Could you check a few things on this model? Use its own coordinates, in mm. Coordinates: 2 decimals unless noted, no trailing zeros. Loops run counter-clockwise (first coordinate to the right, second up) from the corner with the lowest first, then second, coordinate; pieces in that order, holes last.
from build123d import *

# Parameters (mm, degrees)
CYLINDER001_R     = 0.325
CYLINDER001_DEPTH = 10
CYLINDER002_R     = 0.325
CYLINDER002_DEPTH = 10
CYLINDER_R        = 3.75
CYLINDER_DEPTH    = 9.5


with BuildPart() as obj1:
    # Cylinder001 → Cylinder001 (new body)
    with BuildSketch(Plane(origin=(-9, 0, -10), x_dir=(1, 0, 0), z_dir=(0, 0, 1))):
        Circle(CYLINDER001_R)
    extrude(amount=CYLINDER001_DEPTH)


with BuildPart() as fusion:
    # Cone → Cone (revolve)
    with BuildSketch(Plane(origin=(-9, 0, 0), x_dir=(1, 0, 0), z_dir=(0, -1, 0))):
        Polygon((0, 0), (0.325, 0), (1.25, 3), (0, 3), align=None)
    revolve(axis=Axis((-9, 0, 0), (0, 0, 1)))

    # Fusion: union obj1
    add(obj1.part)


with BuildPart() as fusion_1:
    # Fusion placement: moved
    add(fusion.part.moved(Location((10.5, 0, -3))))


with BuildPart() as obj2:
    # Cylinder002 → Cylinder002 (new body)
    with BuildSketch(Plane(origin=(-9, 0, -10), x_dir=(1, 0, 0), z_dir=(0, 0, 1))):
        Circle(CYLINDER002_R)
    extrude(amount=CYLINDER002_DEPTH)


with BuildPart() as fusion001:
    # Cone001 → Cone001 (revolve)
    with BuildSketch(Plane(origin=(-9, 0, 0), x_dir=(1, 0, 0), z_dir=(0, -1, 0))):
        Polygon((0, 0), (0.325, 0), (1.25, 3), (0, 3), align=None)
    revolve(axis=Axis((-9, 0, 0), (0, 0, 1)))

    # Fusion001: union obj2
    add(obj2.part)


with BuildPart() as fusion001_1:
    # Fusion001 placement: moved
    add(fusion001.part.moved(Location((7.5, 0, -3))))


with BuildPart() as fusion002:
    # Cylinder → Cylinder (new body)
    with BuildSketch(Plane.XY):
        Circle(CYLINDER_R)
    extrude(amount=CYLINDER_DEPTH)

    # Fusion002: union Fusion, Fusion001
    add(fusion_1.part)
    add(fusion001_1.part)


solid = fusion002.part
(1) Imagine slicing it at C-C, the plane x = -1.5. Write out the boundary of the cut face in (y, z) (3 decimals).
Answers:
outline: (-3.437, 0) - (-1.25, 0) - (-0.325, -3) - (-0.325, -13) - (0.325, -13) - (0.325, -3) - (1.25, 0) - (3.437, 0) - (3.437, 9.5) - (-3.437, 9.5) - close
(2) For pin 1 (3 mm diameter, centred on x = -2.5, z = 0.5, fed in from +Y); pin 2 (1 mm diameter, centred on x = -1.5, z = 0.5, fed in from -Y), each with a flat end and sliding along its axis, tell me the tip position at first contact or that it passes through.
Answers:
pin 1: stops at y = 3.61
pin 2: stops at y = -3.61
(3) Imagine slicing it at A-A, the plane y = 0. Write out the boundary of the cut face in (x, z) (3 decimals), and give its area (3 significant figures).
Answers:
outline: (-3.75, 0) - (-2.75, 0) - (-1.825, -3) - (-1.825, -13) - (-1.175, -13) - (-1.175, -3) - (-0.25, 0) - (0.25, 0) - (1.175, -3) - (1.175, -13) - (1.825, -13) - (1.825, -3) - (2.75, 0) - (3.75, 0) - (3.75, 9.5) - (-3.75, 9.5) - close
area: 93.7 mm2
(4) We'd pull the mould along X, two halves only. Please class faces 1 (the face through (-3.746, 0.165, 4.684)), 2 (the face through (0, 0, 9.5)), 3 (the face through (-0.84, 0.21, -1.81)): +X half, -X half, draft (parallel to the pull), parting line (faces both ways), or undercut.
Answers:
face 1: parting line
face 2: draft
face 3: undercut
(5) Imagine slicing it at B-B, the plane z = -3.75. Write out the boundary of the cut face in (x, y) (3 decimals).
Answers:
outline: circle Ø0.65 at (-1.5, 0); circle Ø0.65 at (1.5, 0)
(6) I need wall thicknesses on probe 1 along Z at (x, y) = (1.25, -2); probe 2 along Y at (x, z) = (-1.5, -9) (3 decimals); probe 3 along X at (y, z) = (3, 3.5). Which ranges of each line are inside material? Lowest first, please.
Answers:
probe 1: z = 0 to 9.5
probe 2: y = -0.325 to 0.325
probe 3: x = -2.25 to 2.25
(7) Imagine slicing it at D-D, the plane x = 0. Write out the boundary of the cut face in (y, z), and give its area (4 significant figures).
Answers:
outline: (-3.75, 0) - (3.75, 0) - (3.75, 9.5) - (-3.75, 9.5) - close
area: 71.25 mm2
